For this review, take the finished solid that the model builds, in its own axes (mm). A direction names the side the tool comes from. Coordinates: 2 decimals unless noted, no trailing zeros. Write each loop counter-clockwise with the first axis right and the second up, starting at its lowest first coordinate (ties: lowest second). Pieces come first, ordered by that corner, then holes. Notation, with made-up numbers: M 60,2 L 107,2 A22 cw 107,27 Z; hole C -6.5,80 d5. An arc over 180 degrees is marked long. One line per question, with ' | ' between items.
from build123d import *

# Parameters (mm, degrees)
SKICA1_W                  = 54.6
SKICA1_H                  = 54.6
P_IDAT_VYSUNUT_M2_DEPTH   = 3
SKICA14_W                 = 52.6
SKICA14_H                 = 1
P_IDAT_VYSUNUT_M9_DEPTH   = 35
SKICA19_W                 = 7.8
SKICA19_H                 = 7.8
P_IDAT_VYSUNUT_M10_DEPTH  = 38
SKICA20_R                 = 2.4
ODEBRAT_VYSUNUT_M9_DEPTH  = 1.7
ZAOBLIT1_R                = 3
SKICA25_W                 = 32
SKICA25_H                 = 54.6
P_IDAT_VYSUNUT_M12_DEPTH  = 20
SKICA26_W                 = 30
SKICA26_H                 = 52
ODEBRAT_VYSUNUT_M11_DEPTH = 19
SKICA27_W                 = 5.08
SKICA27_H                 = 10.16
ODEBRAT_VYSUNUT_M12_DEPTH = 1
SKICA28_W                 = 9
SKICA28_H                 = 8
ODEBRAT_VYSUNUT_M13_DEPTH = 1
ZAOBLIT3_R                = 4
SKICA29_W                 = 0.5
SKICA29_H                 = 4
ODEBRAT_VYSUNUT_M14_DEPTH = 2
SKICA30_R                 = 0.9
ODEBRAT_VYSUNUT_M15_DEPTH = 2
SKICA31_W                 = 6
SKICA31_H                 = 4
ODEBRAT_VYSUNUT_M16_DEPTH = 2
ZAOBLIT4_R                = 1


with BuildPart() as part:
    # Skica1 → Přidat vysunutím2 (new body)
    with BuildSketch(Plane.XY):
        Rectangle(SKICA1_W, SKICA1_H)
    extrude(amount=P_IDAT_VYSUNUT_M2_DEPTH)

    # Skica14 → Přidat vysunutím9 (add)
    with BuildSketch(Plane.XY.offset(3)):
        Polygon((27.3, 27.3), (-27.3, 27.3), (-27.3, -27.3), (-26.3, -27.3), (-26.3, -26.3), (-26.3, 26.3), (26.3, 26.3), (26.3, -26.3), (26.3, -27.3), (27.3, -27.3), align=None)
        with Locations((0, -26.8)):
            Rectangle(SKICA14_W, SKICA14_H)
    extrude(amount=P_IDAT_VYSUNUT_M9_DEPTH)

    # Skica19 → Přidat vysunutím10 (add)
    with BuildSketch(Plane(origin=(0, 0, 0), x_dir=(-1, 0, 0), z_dir=(0, 0, -1))):
        with Locations((-23.4, 23.4)):
            Rectangle(SKICA19_W, SKICA19_H)
        with Locations((23.4, 23.4)):
            Rectangle(SKICA19_W, SKICA19_H)
        with Locations((-23.4, -23.4)):
            Rectangle(SKICA19_W, SKICA19_H)
        with Locations((23.4, -23.4)):
            Rectangle(SKICA19_W, SKICA19_H)
    extrude(amount=-P_IDAT_VYSUNUT_M10_DEPTH)

    # Skica20 → Odebrat vysunutím9 (cut)
    with BuildSketch(Plane.XY.offset(38)):
        with Locations((-23.4, -23.4)):
            Circle(SKICA20_R)
        with Locations((-23.4, 23.4)):
            Circle(SKICA20_R)
        with Locations((23.400280565, 23.4)):
            Circle(SKICA20_R)
        with Locations((23.400280565, -23.4)):
            Circle(SKICA20_R)
    extrude(amount=-ODEBRAT_VYSUNUT_M9_DEPTH, mode=Mode.SUBTRACT)

    # Zaoblit1
    zaoblit1_edges = [part.edges().sort_by_distance(p)[0] for p in [
        (-19.5, -19.5, 20.5),
        (19.5, 19.5, 20.5),
        (-19.5, 19.5, 20.5),
        (19.5, -19.5, 20.5),
    ]]
    fillet(zaoblit1_edges, radius=ZAOBLIT1_R)

    # Skica25 → Přidat vysunutím12 (add)
    with BuildSketch(Plane(origin=(0, 0, 0), x_dir=(-1, 0, 0), z_dir=(0, 0, -1))):
        Rectangle(SKICA25_W, SKICA25_H)
    extrude(amount=-P_IDAT_VYSUNUT_M12_DEPTH)

    # Skica26 → Odebrat vysunutím11 (cut)
    with BuildSketch(Plane(origin=(0, 0, 0), x_dir=(-1, 0, 0), z_dir=(0, 0, -1))):
        Rectangle(SKICA26_W, SKICA26_H)
    extrude(amount=-ODEBRAT_VYSUNUT_M11_DEPTH, mode=Mode.SUBTRACT)

    # Skica27 → Odebrat vysunutím12 (cut)
    with BuildSketch(Plane.ZY.offset(27.3)):
        with Locations((32.46, 0)):
            Rectangle(SKICA27_W, SKICA27_H)
    extrude(amount=-ODEBRAT_VYSUNUT_M12_DEPTH, mode=Mode.SUBTRACT)

    # Skica28 → Odebrat vysunutím13 (cut)
    with BuildSketch(Plane(origin=(0, 0, 0), x_dir=(-1, 0, 0), z_dir=(0, 0, -1))):
        with Locations((-19.5, 16.940262317)):
            Rectangle(SKICA28_W, SKICA28_H)
    extrude(amount=-ODEBRAT_VYSUNUT_M13_DEPTH, mode=Mode.SUBTRACT)

    # Zaoblit3
    zaoblit3_edges = [part.edges().sort_by_distance(p)[0] for p in [
        (24, 12.940262317, 0.5),
        (24, 20.940262317, 0.5),
    ]]
    fillet(zaoblit3_edges, radius=ZAOBLIT3_R - 0.0001)  # a hair under: the kernel refuses the full size

    # Skica29 → Odebrat vysunutím14 (cut)
    with BuildSketch(Plane(origin=(-15, 0, 0), x_dir=(0, 0, -1), z_dir=(1, 0, 0))):
        with Locations((-0.75, 19)):
            Rectangle(SKICA29_W, SKICA29_H)
        with Locations((-0.83, -19)):
            Rectangle(SKICA29_W, SKICA29_H)
    extrude(amount=-ODEBRAT_VYSUNUT_M14_DEPTH, mode=Mode.SUBTRACT)

    # Skica30 → Odebrat vysunutím15 (cut)
    with BuildSketch(Plane(origin=(0, 0, 1), x_dir=(-1, 0, 0), z_dir=(0, 0, -1))):
        with Locations((-20, 16.940262317)):
            Circle(SKICA30_R)
    extrude(amount=-ODEBRAT_VYSUNUT_M15_DEPTH, mode=Mode.SUBTRACT)

    # Skica31 → Odebrat vysunutím16 (cut)
    with BuildSketch(Plane(origin=(0, 0, 19), x_dir=(-1, 0, 0), z_dir=(0, 0, -1))):
        with Locations((-12, 24)):
            Rectangle(SKICA31_W, SKICA31_H)
    extrude(amount=-ODEBRAT_VYSUNUT_M16_DEPTH, mode=Mode.SUBTRACT)

    # Zaoblit4
    zaoblit4_edges = [part.edges().sort_by_distance(p)[0] for p in [
        (9, 22, 19.5),
    ]]
    fillet(zaoblit4_edges, radius=ZAOBLIT4_R)


solid = part.part
1) Insertion check: pin 1 Ø1 at (x, y) = (-18, 15) entering from +Z; pin 2 Ø6 at (x, y) = (-10.5, 14) entering from -Z; pin 3 Ø1.4 at (x, y) = (-22.5, -23.5) entering from +Z. Each pin has a flat end and moves straight along its axis. Give the tip position at first contact, or say it passes through.
Responses:
pin 1: z = 3 | pin 2: z = 19 | pin 3: z = 36.3
2) To check wall thickness, follow line 1 along X through (y, z) = (12, 6.5); line 2 along Y through (x, z) = (17, 32.5); line 3 along Y through (x, z) = (-23, 23.5). State the ranges of each line that lie inside material, in increasing order. Write a range as [from, to].
Responses:
line 1: [-27.3, -26.3], [-16, -15], [15, 16], [26.3, 27.3] | line 2: [-27.3, -26.3], [26.3, 27.3] | line 3: [-27.3, -19.5], [19.5, 27.3]
3) We need section A-A on x = 14. State the section outline as (y, z) points.
Responses:
outline: M -27.3,0 L -26,0 L -26,19 L 22,19 L 22,20 L -26.3,20 L -26.3,38 L -27.3,38 Z; M 26,0 L 27.3,0 L 27.3,38 L 26.3,38 L 26.3,20 L 26,20 Z
4) The part is to be moulded in two halves that separate along Y. For faces 1 (the flat face through (27.3, 0, 19)), 2 (the flat face through (-16, 19, 0.5)), say which applies: +Y half, -Y half, draft (parallel to the pull), parting line (faces both ways), or undercut.
Responses:
face 1: draft | face 2: undercut
5) Machinability: for faces 3 (the flat face through (0, 26, 10)), 4 (the flat face through (-27.3, 0, 19)), 5 (the flat face through (-24, -19.5, 20)), 6 (the flat face through (-16, 19, 1)), which of the approach directions +Z, -Z, +X, -X, +Y, -Y give a long, thin tool a straight path to every point of the face, cutting with its end or side? Answer none if there is none.
Responses:
face 3: -Z | face 4: +Z, -Z, -X, +Y, -Y | face 5: +Z | face 6: none
6) We need section D-D on z = 33.5. State the section outline as (x, y) points.
Responses:
outline: M -27.3,-27.3 L 27.3,-27.3 L 27.3,27.3 L -27.3,27.3 L -27.3,5.08 L -26.3,5.08 L -26.3,19.5 L -22.5,19.5 A3 ccw -19.5,22.5 L -19.5,26.3 L 19.5,26.3 L 19.5,22.5 A3 ccw 22.5,19.5 L 26.3,19.5 L 26.3,-19.5 L 22.5,-19.5 A3 ccw 19.5,-22.5 L 19.5,-26.3 L -19.5,-26.3 L -19.5,-22.5 A3 ccw -22.5,-19.5 L -26.3,-19.5 L -26.3,-5.08 L -27.3,-5.08 Z
7) We need section C-C on y = -23.4. State the section outline as (x, z) points.
Responses:
outline: M -27.3,0 L -15,0 L -15,19 L 15,19 L 15,0 L 27.3,0 L 27.3,38 L 25.8,38 L 25.8,36.3 L 21,36.3 L 21,38 L 19.5,38 L 19.5,3 L 16,3 L 16,20 L -16,20 L -16,3 L -19.5,3 L -19.5,38 L -21,38 L -21,36.3 L -25.8,36.3 L -25.8,38 L -27.3,38 Z
8) We need section B-B on z = 7.5. State the section outline as (x, y) points.
Responses:
outline: M -27.3,-27.3 L 27.3,-27.3 L 27.3,27.3 L -27.3,27.3 Z; hole M -26.3,-19.5 L -22.5,-19.5 A3 cw -19.5,-22.5 L -19.5,-26.3 L -16,-26.3 L -16,26.3 L -19.5,26.3 L -19.5,22.5 A3 cw -22.5,19.5 L -26.3,19.5 Z; hole M -15,-26 L 15,-26 L 15,26 L -15,26 Z; hole M 16,-26.3 L 19.5,-26.3 L 19.5,-22.5 A3 cw 22.5,-19.5 L 26.3,-19.5 L 26.3,19.5 L 22.5,19.5 A3 cw 19.5,22.5 L 19.5,26.3 L 16,26.3 Z
